```python
from build123d import *

# Parameters (mm, degrees)
SKETCH_2_W          = 105
SKETCH_2_H          = 65
EXTRUDE_1_DEPTH     = 110
SKETCH_3_R          = 7
SKETCH_3_R_2        = 8
CUT_EXTRUDE_1_DEPTH = 50
SKETCH_4_R          = 20.5
CUT_EXTRUDE_2_DEPTH = 156.503215401


with BuildPart() as part:
    # 草图2 → 凸台-拉伸1 (new body)
    with BuildSketch(Plane.XY):
        Rectangle(SKETCH_2_W, SKETCH_2_H)
    extrude(amount=-EXTRUDE_1_DEPTH)

    # 草图3 → 切除-拉伸1 (cut)
    with BuildSketch(Plane.XY):
        with Locations((-32.5, -0.5)):
            Circle(SKETCH_3_R)
        with Locations((31.5, 0)):
            Circle(SKETCH_3_R)
        Circle(SKETCH_3_R_2)
    extrude(amount=-CUT_EXTRUDE_1_DEPTH, mode=Mode.SUBTRACT)

    # 草图4 → 切除-拉伸2 (cut, through all)
    with BuildSketch(Plane(origin=(52.5, 0, 0), x_dir=(0, 0, -1), z_dir=(1, 0, 0))):
        with Locations(Location((83, -7.5, 0), (0, 0, 90))):
            Circle(SKETCH_4_R)
    extrude(amount=-CUT_EXTRUDE_2_DEPTH, mode=Mode.SUBTRACT)


solid = part.part
```
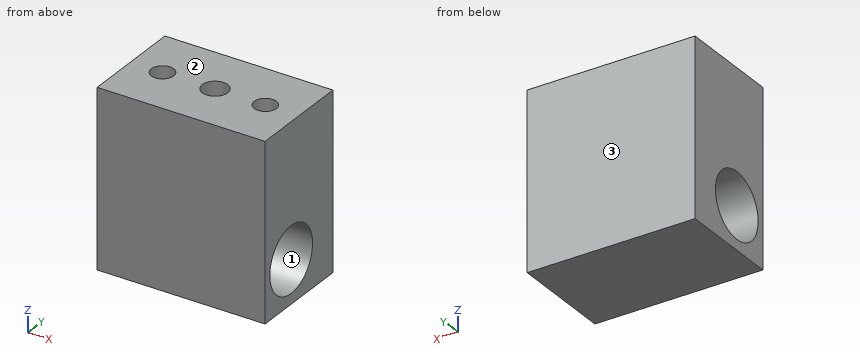
Build history of the part. All positions in model axes, mm. Face numbers are marked on the shaded views. Round coordinates to 2 decimals unless told otherwise and drop trailing zeros. Write each loop counter-clockwise with the first axis right and the second up, starting at its lowest first coordinate (ties: lowest second). Pieces come first, ordered by that corner, then holes. Notation, with made-up numbers: (24, 69) - (31, 69) arc R15 ccw to (31, 74) - close; hole circle Ø10 at (32.25, 16). An arc over 180 degrees is marked (long way). Write each question's results on one line, items separated by ' | '. Start each with the question number.
Item 1: Saw through at D-D (z = -44). Write the cut outline in (x, y), and give its area (3 significant figures).
Item 2: Wall check: L1, parallel to Z at x = -41.5, y = -7; L2, parallel to Y at x = -32, z = -11; L3, parallel to Z at x = -39, y = 10. Give the ranges that are in metal, low to high. Write a range as [from, to].
Item 3: Saw through at C-C (y = -24.5). Write the cut outline in (x, z).
Item 4: Saw through at B-B (z = -65.5). Write the cut outline in (x, y).
Item 5: Saw through at A-A (x = 0). Write the cut outline in (y, z).
Item 6: Mould opens along Y. For the marked faces 1, 2 and 3 say: pulls with the +Y half, pulls with the -Y half, needs draft (parallel to the pull), parting line crosses it, or undercut.
Item 7: Drop a flat-ended pin along its axis: P1, Ø4, axis at x = 34, y = 0.5, coming from the +Z side. Give the stop position or say it passes through.
Results are:
1) outline: (-52.5, -32.5) - (52.5, -32.5) - (52.5, 32.5) - (-52.5, 32.5) - close; hole circle Ø14 at (-32.5, -0.5); hole circle Ø16 at (0, 0); hole circle Ø14 at (31.5, 0) | area: 6,320 mm²
2) L1: z = [-110, -103.49], [-62.51, 0] | L2: y = [-32.5, -7.48], [6.48, 32.5] | L3: z = [-110, -93.68], [-72.32, 0]
3) outline: (-52.5, -110) - (52.5, -110) - (52.5, -94.46) - (-52.5, -94.46) - close; (-52.5, -71.54) - (52.5, -71.54) - (52.5, 0) - (-52.5, 0) - close
4) outline: (-52.5, -32.5) - (52.5, -32.5) - (52.5, -18.18) - (-52.5, -18.18) - close; (-52.5, 3.18) - (52.5, 3.18) - (52.5, 32.5) - (-52.5, 32.5) - close
5) outline: (-32.5, -110) - (32.5, -110) - (32.5, 0) - (8, 0) - (8, -50) - (-8, -50) - (-8, 0) - (-32.5, 0) - close; hole circle Ø41 at (-7.5, -83)
6) face 1: undercut | face 2: needs draft | face 3: pulls with the +Y half
7) P1: stops at z = -50
